Source: CAD feature listing. Evaluate the final solid. Frame: model axes, mm. Face numbers are marked on the shaded views. A direction names the side the tool comes from. Give positions to 0.01 mm unless a question says otherwise; leave off trailing zeros. Order: outer loops, then holes, each group sorted by start corner. A loop starts at its lowest first (then second) coordinate and runs counter-clockwise, first axis right, second up.
from build123d import *

# Parameters (mm, degrees)
SKETCH1_R           = 27.5
BOSS_EXTRUDE1_DEPTH = 12.7
BOSS_EXTRUDE2_START = -12.7
SKETCH2_R           = 2
BOSS_EXTRUDE2_DEPTH = 12.7
SKETCH7_R           = 2
CUT_EXTRUDE4_DEPTH  = 85
SKETCH8_R           = 2.5
SKETCH8_W           = 50.8
SKETCH8_H           = 50.8
CUT_EXTRUDE5_DEPTH  = 12.7
SKETCH9_R           = 1.25
CUT_EXTRUDE6_DEPTH  = 12.7
SKETCH10_R          = 3.75
CUT_EXTRUDE7_DEPTH  = 10.7
SKETCH11_R          = 3.75
CUT_EXTRUDE8_DEPTH  = 10.7


with BuildPart() as part:
    # Sketch1 → Boss-Extrude1 (new body)
    with BuildSketch(Plane.XY):
        with BuildLine():
            Line((30.675000233, 40), (30.675000233, -40))
            ThreePointArc((30.675000233, -40), (0, -70.675000233), (-30.675000233, -40))
            Line((-30.675000233, -40), (-30.675000233, 40))
            ThreePointArc((-30.675000233, 40), (0, 70.675000233), (30.675000233, 40))
        make_face()
        with Locations((0, -40)):
            Circle(SKETCH1_R, mode=Mode.SUBTRACT)
        with Locations(Location((0, 40, 0), (0, 0, 180))):
            Circle(SKETCH1_R, mode=Mode.SUBTRACT)
    extrude(amount=BOSS_EXTRUDE1_DEPTH)

    # Sketch2 → Boss-Extrude2 (add)
    with BuildSketch(Plane.XY.offset(12.7).offset(BOSS_EXTRUDE2_START)):
        with BuildLine():
            Line((-30.675000233, 40), (-30.675000233, -40))
            ThreePointArc((-30.675000233, -40), (0, -70.675000233), (30.675000233, -40))
            Line((30.675000233, -40), (30.675000233, 40))
            ThreePointArc((30.675000233, 40), (0, 70.675000233), (-30.675000233, 40))
        make_face()
        with Locations((20.784609691, 52)):
            Circle(SKETCH2_R, mode=Mode.SUBTRACT)
        with Locations((-20.784609691, 52)):
            Circle(SKETCH2_R, mode=Mode.SUBTRACT)
        with Locations((-20.784609691, -52)):
            Circle(SKETCH2_R, mode=Mode.SUBTRACT)
        with Locations((20.784609691, -52)):
            Circle(SKETCH2_R, mode=Mode.SUBTRACT)
    extrude(amount=BOSS_EXTRUDE2_DEPTH)

    # Sketch7 → Cut-Extrude4 (cut)
    with BuildSketch(Plane.ZY.offset(30.675000233)):
        with Locations(Location((6.35, 0, 0), (0, 0, 270))):
            Circle(SKETCH7_R)
    extrude(amount=-CUT_EXTRUDE4_DEPTH, mode=Mode.SUBTRACT)

    # Sketch8 → Cut-Extrude5 (cut)
    with BuildSketch(Plane.XY.offset(12.7)):
        with Locations((0, 44.4)):
            Circle(SKETCH8_R)
        with Locations((0, -44.4)):
            Circle(SKETCH8_R)
        Rectangle(SKETCH8_W, SKETCH8_H)
    extrude(amount=-CUT_EXTRUDE5_DEPTH, mode=Mode.SUBTRACT)

    # Sketch9 → Cut-Extrude6 (cut)
    with BuildSketch(Plane(origin=(0, 0, 0), x_dir=(-1, 0, 0), z_dir=(0, 0, -1))):
        with Locations((-25.4, 25.4)):
            Circle(SKETCH9_R)
        with Locations((25.4, 25.4)):
            Circle(SKETCH9_R)
        with Locations((25.4, -25.4)):
            Circle(SKETCH9_R)
        with Locations((-25.4, -25.4)):
            Circle(SKETCH9_R)
    extrude(amount=-CUT_EXTRUDE6_DEPTH, mode=Mode.SUBTRACT)

    # Sketch10 → Cut-Extrude7 (cut)
    with BuildSketch(Plane(origin=(0, 0, 0), x_dir=(-1, 0, 0), z_dir=(0, 0, -1))):
        with Locations((-20.784609691, 52)):
            Circle(SKETCH10_R)
        with Locations(Location((20.784609691, 52, 0), (0, 0, 180))):
            Circle(SKETCH10_R)
        with Locations((20.784609691, -52)):
            Circle(SKETCH10_R)
        with Locations(Location((-20.784609691, -52, 0), (0, 0, 180))):
            Circle(SKETCH10_R)
    extrude(amount=-CUT_EXTRUDE7_DEPTH, mode=Mode.SUBTRACT)

    # Sketch11 → Cut-Extrude8 (cut)
    with BuildSketch(Plane.XY.offset(12.7)):
        with Locations((0, 44.4)):
            Circle(SKETCH11_R)
        with Locations((0, -44.4)):
            Circle(SKETCH11_R)
    extrude(amount=-CUT_EXTRUDE8_DEPTH, mode=Mode.SUBTRACT)


solid = part.part
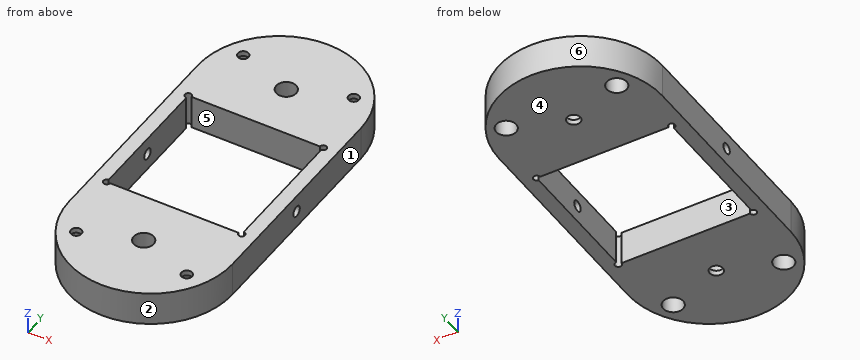
1) Pull-direction query (X, two-part tool) for the marked faces 1, 2, 3 and 4; classes: +X half, -X half, draft (parallel to the pull), parting line (faces both ways), or undercut.
Checks:
face 1: +X half
face 2: parting line
face 3: undercut
face 4: draft
2) Section query B-B on x = 0. Output: boundary loops of the cut face in (y, z) (3 decimals), and give its area (3 significant figures).
Checks:
outline: (-70.675, 0) - (-46.9, 0) - (-46.9, 2) - (-48.15, 2) - (-48.15, 12.7) - (-70.675, 12.7) - close; (-41.9, 0) - (-25.4, 0) - (-25.4, 12.7) - (-40.65, 12.7) - (-40.65, 2) - (-41.9, 2) - close; (25.4, 0) - (41.9, 0) - (41.9, 2) - (40.65, 2) - (40.65, 12.7) - (25.4, 12.7) - close; (46.9, 0) - (70.675, 0) - (70.675, 12.7) - (48.15, 12.7) - (48.15, 2) - (46.9, 2) - close
area: 969 mm2
3) First-contact query: pin 1 Ø5 at (x, z) = (-19, 9) entering from -Y; pin 2 Ø2 at (x, y) = (-1.5, 44) entering from +Z; pin 3 Ø2.5 at (y, z) = (0, 6.35) entering from -X; pin 4 Ø6 at (y, z) = (-49.5, 4) entering from +X. Flat tips, straight axial feed; report the tip coordinate or a pass-through.
Checks:
pin 1: stops at y = -65.86
pin 2: stops at z = 2
pin 3: passes through
pin 4: stops at x = 29.98
4) Section query C-C on y = -52. Output: boundary loops of the cut face in (x, z).
Checks:
outline: (-28.23, 0) - (-24.53, 0) - (-24.53, 10.7) - (-22.78, 10.7) - (-22.78, 12.7) - (-28.23, 12.7) - close; (-18.78, 10.7) - (-17.03, 10.7) - (-17.03, 0) - (17.03, 0) - (17.03, 10.7) - (18.78, 10.7) - (18.78, 12.7) - (-18.78, 12.7) - close; (22.78, 10.7) - (24.53, 10.7) - (24.53, 0) - (28.23, 0) - (28.23, 12.7) - (22.78, 12.7) - close
5) Ray query, L1, parallel to Y at x = 0, z = 1.25 (3 decimals); L2, parallel to X at y = 3, z = 11.5 (3 decimals); L3, parallel to Y at x = 18, z = 3. Return the intervals inside material, ascending.
Checks:
L1: y = -70.675 to -46.9, -41.9 to -25.4, 25.4 to 41.9, 46.9 to 70.675
L2: x = -30.675 to -25.4, 25.4 to 30.675
L3: y = -64.84 to -54.51, -49.49 to -25.4, 25.4 to 49.49, 54.51 to 64.84
6) Reachability of the marked faces 5 and 6 from +Z, -Z, +X, -X, +Y, -Y: full face, straight path, thin tool, end or side. Return the list, or none.
Checks:
face 5: +Z, -Z
face 6: +Z, -Z, +Y
7) Section query A-A on z = 6.35. Output: boundary loops of the cut face in (x, y) (3 decimals).
Checks:
outline: (-30.675, -40) arc R30.675 ccw to (30.675, -40) - (30.675, -2) - (25.4, -2) - (25.4, -24.15) arc R1.25 cw (long way) to (24.15, -25.4) - (-24.15, -25.4) arc R1.25 cw (long way) to (-25.4, -24.15) - (-25.4, -2) - (-30.675, -2) - close; (-30.675, 2) - (-25.4, 2) - (-25.4, 24.15) arc R1.25 cw (long way) to (-24.15, 25.4) - (24.15, 25.4) arc R1.25 cw (long way) to (25.4, 24.15) - (25.4, 2) - (30.675, 2) - (30.675, 40) arc R30.675 ccw to (-30.675, 40) - close; hole circle Ø7.5 at (-20.785, -52); hole circle Ø7.5 at (-20.785, 52); hole circle Ø7.5 at (0, -44.4); hole circle Ø7.5 at (0, 44.4); hole circle Ø7.5 at (20.785, -52); hole circle Ø7.5 at (20.785, 52)
8) Section query D-D on y = 17. Output: boundary loops of the cut face in (x, z) (3 decimals), and give its area (3 significant figures).
Checks:
outline: (-30.675, 0) - (-25.4, 0) - (-25.4, 12.7) - (-30.675, 12.7) - close; (25.4, 0) - (30.675, 0) - (30.675, 12.7) - (25.4, 12.7) - close
area: 134 mm2
